```python
from build123d import *

# Parameters (mm, degrees)
SKETCH039_R      = 3.5
EXTRUDE058_DEPTH = 5
SKETCH029_W      = 23
SKETCH029_H      = 90
EXTRUDE028_DEPTH = 10


with BuildPart() as union_centro_arriba:
    # Sketch039 → Extrude058 (new body)
    with BuildSketch(Plane(origin=(0, 0, 0), x_dir=(0, -1, 0), z_dir=(-1, 0, 0))):
        with BuildLine():
            ThreePointArc((2.488294, 145.254171), (-2.511706, 150.254171), (-7.511706, 145.254171))
            Line((-7.511706, 145.254171), (-7.511706, 127.933024))
            ThreePointArc((-7.511706, 127.933024), (-2.511706, 122.933024), (2.488294, 127.933024))
            Line((2.488294, 145.254171), (2.488294, 127.933024))
        make_face()
        with Locations((-2.820375, 145.089175)):
            Circle(SKETCH039_R, mode=Mode.SUBTRACT)
    extrude(amount=EXTRUDE058_DEPTH)


with BuildPart() as union_centro_arriba_1:
    # Extrude058 placement: moved
    add(union_centro_arriba.part.moved(Location((55, -0.03, 0))))


with BuildPart() as union_centro_arriba001:
    # Link022 base: copy of union centro_arriba
    add(union_centro_arriba_1.part)


with BuildPart() as union_centro_arriba001_1:
    # Link022 placement: moved
    add(union_centro_arriba001.part.moved(Location((18, 0, 0))))


with BuildPart() as obj1:
    # Sketch029 → Extrude028 (new body)
    with BuildSketch(Plane.XZ):
        with Locations((68.040845, 88.110787)):
            Rectangle(SKETCH029_W, SKETCH029_H)
        Polygon((60.680845, 57.610787), (75.403277, 66.110787), (75.403277, 49.110787), align=None, mode=Mode.SUBTRACT)
        Polygon((60.678413, 65.110787), (60.678413, 82.110787), (75.400845, 73.610787), align=None, mode=Mode.SUBTRACT)
        Polygon((60.680845, 89.610787), (75.403277, 98.110787), (75.403277, 81.110787), align=None, mode=Mode.SUBTRACT)
        Polygon((60.678413, 97.110787), (60.678413, 114.110787), (75.400845, 105.610787), align=None, mode=Mode.SUBTRACT)
        Polygon((60.680845, 121.610787), (75.403277, 130.110787), (75.403277, 113.110787), align=None, mode=Mode.SUBTRACT)
    extrude(amount=EXTRUDE028_DEPTH)


with BuildPart() as obj1_1:
    # Extrude028 placement: moved
    add(obj1.part.moved(Location((-6.55, 7.5, -5.11))))

    # Fusion: union union centro_arriba, union centro_arriba001
    add(union_centro_arriba_1.part)
    add(union_centro_arriba001_1.part)


solid = obj1_1.part
```
Verification items for the finished model (mm, model axes). A direction names the side the tool comes from. Round coordinates to 2 decimals unless told otherwise and drop trailing zeros. Order: outer loops, then holes, each group sorted by start corner. A loop starts at its lowest first (then second) coordinate and runs counter-clockwise, first axis right, second up. Notation, with made-up numbers: (-30, 61) -> (-10, 61) arc R10 cw to (-10, 75) -> close; hole circle Ø8 at (31.5, 34.25). An arc over 180 degrees is marked (long way). Put each result on its own line as item: value. Start each with the question number.
(1) Material ranges on line 1 along Z through (x, y) = (58.75, 3); line 2 along Z through (x, y) = (60, -0.75); line 3 along X through (y, z) = (3, 100), recorded low to high.
(2) Depth check by flat-ended pin: pin 1 Ø4 at (x, z) = (51.5, 139.5) entering from +Y; pin 2 Ø12 at (x, z) = (57.5, 75) entering from -Y; pin 3 Ø5 at (y, z) = (1, 139) entering from -X. Enter the tip coordinate at first touch or a pass-through.
(3) Tool access check on faces 4 (the face through (52.54, 3.25, 148.56)), 5 (the face through (61.6, 2.57, 112.19)). Record the directions out of +Z, -Z, +X, -X, +Y, -Y that give a thin tool (end or side, any length) a straight path to the whole face; none if there is none.
(4) Section check C-C (y = 3). State how many separate pieces and enclosed holes the cut face has, then the cut area to 3 significant figures.
(5) Section check B-B (x = 57.5). Enter the section's corners in (y, z), then the cut area to 3 significant figures.
(6) Draft check along Z on faces 1 (the face through (61, 3, 38.001)), 2 (the face through (53, -2.518, 137)), 3 (the face through (61.39, 2.57, 72.81)). Enter one of: +Z half, -Z half, draft (parallel to the pull), parting line (faces both ways), or undercut.
(7) Section check A-A (z = 65). Enter the section's corners in (x, y), then the cut area to 3 significant figures.
Completed:
1. line 1: z = 38 to 49.83, 55.17 to 62.67, 74.33 to 81.83, 87.17 to 94.67, 106.33 to 113.83, 119.17 to 128
1. line 2: z = 38 to 49.11, 55.89 to 63.39, 73.61 to 81.11, 87.89 to 95.39, 105.61 to 113.11, 119.89 to 128
1. line 3: x = 49.99 to 54.13, 67.98 to 72.99
2. pin 1: stops at y = 7.48
2. pin 2: stops at y = -2.5
2. pin 3: stops at x = 50
3. face 4: +X, -X
3. face 5: +Y, -Y
4. separate pieces: 3
4. enclosed holes: 5
4. area: 1,600 mm2
5. outline: (-2.5, 38) -> (7.5, 38) -> (7.5, 50.56) -> (-2.5, 50.56) -> close; (-2.5, 54.45) -> (7.5, 54.45) -> (7.5, 61.95) -> (-2.5, 61.95) -> close; (-2.5, 75.05) -> (7.5, 75.05) -> (7.5, 82.56) -> (-2.5, 82.56) -> close; (-2.5, 86.45) -> (7.5, 86.45) -> (7.5, 93.95) -> (-2.5, 93.95) -> close; (-2.5, 107.05) -> (7.5, 107.05) -> (7.5, 114.56) -> (-2.5, 114.56) -> close; (-2.5, 118.45) -> (7.5, 118.45) -> (7.5, 128) -> (-2.5, 128) -> close
5. area: 521 mm2
6. face 1: -Z half
6. face 2: draft
6. face 3: undercut
7. outline: (49.99, -2.5) -> (54.13, -2.5) -> (54.13, 7.5) -> (49.99, 7.5) -> close; (62.79, -2.5) -> (72.99, -2.5) -> (72.99, 7.5) -> (62.79, 7.5) -> close
7. area: 143 mm2
